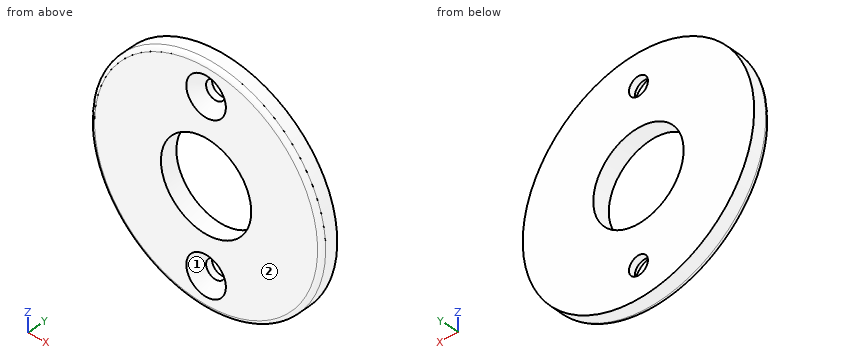
from build123d import *

# Parameters (mm, degrees)
CSK_SLOT_FOR_M4_COUNTERSUNK_FLAT_HEA_2_COUNT = 2
CSK_SLOT_FOR_M4_COUNTERSUNK_FLAT_HEA_2_PITCH = 40
FILLET1_R                                    = 2
FILLET2_R                                    = 1
SKETCH5_R                                    = 32.94079545
CUT_EXTRUDE2_DEPTH                           = 10
SKETCH6_R                                    = 10.732050808
CUT_EXTRUDE3_DEPTH                           = 10


with BuildPart() as part:
    # Sketch1 → Revolve1 (revolve)
    with BuildSketch(Plane.XY, mode=Mode.PRIVATE) as revolve1_sk:
        Polygon((-27.5, 0), (-27.5, 4), (-13, 4), (-13, 8), (-11, 8), (-11, 3), (0, 3), (0, 0), align=None)
    revolve(revolve1_sk.sketch.rotate(Axis((0, 0, 0), (0, -1, 0)), 270), axis=Axis((0, 0, 0), (0, -1, 0)))

    # Sketch3 → CSK SLOT for M4 Countersunk Flat Head Screw1 (revolve, cut)
    with BuildSketch(Plane(origin=(0, 0, 20), x_dir=(0, 0, -1), z_dir=(1, 0, 0))):
        Polygon((0, 0), (0, 4), (2.25, 4), (2.25, 2.45), (4.7, 0), align=None)
    csk_slot_for_m4_countersunk_flat_head_sc = revolve(axis=Axis((0, -6.35, 20), (0, 1, 0)), mode=Mode.SUBTRACT)

    # CSK SLOT for M4 Countersunk Flat Hea 2: CSK SLOT for M4 Countersunk Flat Head Screw1 ×2
    with Locations(*[(0, 0, -i * CSK_SLOT_FOR_M4_COUNTERSUNK_FLAT_HEA_2_PITCH) for i in range(1, CSK_SLOT_FOR_M4_COUNTERSUNK_FLAT_HEA_2_COUNT)]):
        add(csk_slot_for_m4_countersunk_flat_head_sc, mode=Mode.SUBTRACT)

    # Fillet1
    fillet1_edges = [part.edges().sort_by_distance(p)[0] for p in [
        (0, 3, -11),
    ]]
    fillet(fillet1_edges, radius=FILLET1_R)

    # Fillet2
    fillet2_edges = [part.edges().sort_by_distance(p)[0] for p in [
        (0, 0, -27.5),
    ]]
    fillet(fillet2_edges, radius=FILLET2_R)

    # Sketch5 → Cut-Extrude2 (cut)
    with BuildSketch(Plane(origin=(0, 4, 0), x_dir=(1, 0, 0), z_dir=(0, 1, 0))):
        Circle(SKETCH5_R)
    extrude(amount=CUT_EXTRUDE2_DEPTH, mode=Mode.SUBTRACT)

    # Sketch6 → Cut-Extrude3 (cut)
    with BuildSketch(Plane(origin=(0, 4, 0), x_dir=(1, 0, 0), z_dir=(0, 1, 0))):
        with Locations(Location((0, 0, 0), (0, 0, 270))):
            Circle(SKETCH6_R)
    extrude(amount=-CUT_EXTRUDE3_DEPTH, mode=Mode.SUBTRACT)


solid = part.part
The listing builds one solid part. Answer for the finished solid, in the listing's coordinates (mm). Face numbers are marked on the shaded views. Give positions to 0.01 mm unless a question says otherwise; leave off trailing zeros. Order: outer loops, then holes, each group sorted by start corner. A loop starts at its lowest first (then second) coordinate and runs counter-clockwise, first axis right, second up. Notation, with made-up numbers: (0.5, 78) - (8.5, 78) arc R12 ccw to (8.5, 98) - close; hole circle Ø6 at (9.5, 68.25). An arc over 180 degrees is marked (long way). One line per item, written item: value. Start each with the question number.
1) Find the intervals of material crossed by L1, parallel to X at y = 3.15, z = 0; L2, parallel to Z at x = 2.5, y = 1.15; L3, parallel to X at y = 2.45, z = -1.5, in increasing order.
2) The mould has two halves that part along Z. Classify the marked faces 1 and 2: released by +Z, released by -Z, zero draft, split by the parting line, or undercut.
3) A cutting plane is placed at B-B on x = 0. Give the vertices of the cut face in (y, z).
4) Given pin 1 Ø1.5 at (x, y) = (3.5, 3) entering from -Z; pin 2 Ø1 at (y, z) = (1, -11) entering from -X; pin 3 Ø1.5 at (y, z) = (3.5, -8.5) entering from +X; pin 4 Ø4 at (x, z) = (0, 20) entering from +Y, each flat-ended and moving along its own axis, determine where each tip first touches the part or whether it passes through.
5) A cutting plane is placed at A-A on z = 0. Give the vertices of the cut face in (x, y).
Answer sheet:
1. L1: x = -27.5 to -10.73, 10.73 to 27.5
1. L2: z = -27.39 to -22.52, -17.48 to -10.44, 10.44 to 17.48, 22.52 to 27.39
1. L3: x = -27.46 to -10.63, 10.63 to 27.46
2. face 1: undercut
2. face 2: zero draft
3. outline: (0, -26.5) arc R1 ccw to (1, -27.5) - (4, -27.5) - (4, -22.25) - (2.45, -22.25) - (0, -24.7) - close; (0, -15.3) - (2.45, -17.75) - (4, -17.75) - (4, -10.73) - (0, -10.73) - close; (0, 10.73) - (4, 10.73) - (4, 17.75) - (2.45, 17.75) - (0, 15.3) - close; (0, 24.7) - (2.45, 22.25) - (4, 22.25) - (4, 27.5) - (1, 27.5) arc R1 ccw to (0, 26.5) - close
4. pin 1: stops at z = -27.36
4. pin 2: stops at x = -25.42
4. pin 3: stops at x = 26.39
4. pin 4: passes through
5. outline: (-27.5, 1) arc R1 ccw to (-26.5, 0) - (-10.73, 0) - (-10.73, 4) - (-27.5, 4) - close; (10.73, 0) - (26.5, 0) arc R1 ccw to (27.5, 1) - (27.5, 4) - (10.73, 4) - close
